Autodesk Inventor part; units mm, degrees
ref_plane "YZ Plane" through (0, 0, 0) normal (1, 0, 0) x (0, 1, 0)
ref_plane "XZ Plane" through (0, 0, 0) normal (0, 1, 0) x (-1, 0, 0)
ref_plane "XY Plane" through (0, 0, 0) normal (0, 0, 1) x (1, 0, 0)
sketch "スケッチ1" plane through (0, 0, 0) normal (0, 1, 0) x (-1, 0, 0)
  circle A0 centre (0, 0) radius 25
  circle A1 centre (0, 0) radius 30
  dimension "d0" = 50
  dimension "d1" = 60
extrude "押し出し1" add sketch "スケッチ1" along normal blind 60
sketch "スケッチ2" plane through (0, 0, 0) normal (0, 0, 1) x (1, 0, 0)
  line L0 (-5, 30.9364) -> (5, 30.9364)
  line L1 (5, 30.9364) -> (5, 22.9364)
  line L2 (5, 22.9364) -> (-5, 22.9364)
  line L3 (-5, 22.9364) -> (-5, 30.9364)
  line L4 (-5, 30.9364) -> (5, 22.9364) construction
  line L5 (5, 30.9364) -> (-5, 22.9364) construction
  point P0 (0, 0)
  point P1 (0, 26.9364)
  dimension "d4" = 10
  dimension "d5" = 8
extrude "押し出し2" cut sketch "スケッチ2" along normal mid plane 60
sketch "スケッチ3" plane through (0, 0, 0) normal (0, 0, 1) x (1, 0, 0)
  point P0 (0, 0)
sketch "スケッチ4" plane through (0, 0, 0) normal (0, 0, 1) x (1, 0, 0)
  line L0 (4, -5) -> (-4, -5)
  line L1 (-4, -5) -> (-4, 5)
  line L2 (-4, 5) -> (4, 5)
  line L3 (4, 5) -> (4, -5)
  line L4 (4, -5) -> (-4, 5) construction
  line L5 (-4, -5) -> (4, 5) construction
  point P0 (0, 0)
  dimension "d8" = 8
  dimension "d9" = 10
extrude "押し出し3" cut sketch "スケッチ4" along normal mid plane 60
properties part number "pipe"
Can you work these out from the model? Positions are in its coordinate system, mm. A direction names the side the tool comes from. Give positions to 0.01 mm unless a question says otherwise; leave off trailing zeros. Loops run counter-clockwise (first coordinate to the right, second up) from the corner with the lowest first, then second, coordinate; pieces in that order, holes last. Notation, with made-up numbers: (68.25, 73) -> (74.25, 73) arc R29 cw to (74.25, 97) -> close; hole circle Ø1 at (13.5, 53). An arc over 180 degrees is marked (long way). Use one line per item in the form item = value.
1) If we section it at C-C (x = -9): Please give me the cut outline in (y, z), plus the area to 3 significant figures.
Answers:
outline = (0, -28.62) -> (60, -28.62) -> (60, -23.32) -> (0, -23.32) -> close; (0, 23.32) -> (60, 23.32) -> (60, 28.62) -> (0, 28.62) -> close
area = 635 mm²
2) Will these pins go through, and if not, where does the flat tip stop? pin 1 (3 mm diameter, centred on x = -1, z = -27, fed in from -Y); pin 2 (12 mm diameter, centred on x = 22.5, y = 20, fed in from -Z); pin 3 (2 mm diameter, centred on y = 7.5, z = -4, fed in from +X); pin 4 (12 mm diameter, centred on y = 38.5, z = 4, fed in from -X).
Answers:
pin_1 = 5
pin_2 = -25.05
pin_3 = 29.85
pin_4 = -30
3) If we section it at D-D (y = 33): Please give me the cut outline in (x, z).
Answers:
outline = circle Ø60 at (0, 0); hole circle Ø50 at (0, 0)
4) If we section it at A-A (x = 0): Please give me the cut outline in (y, z), plus the area to 3 significant figures.
Answers:
outline = (5, -30) -> (22.94, -30) -> (22.94, -25) -> (5, -25) -> close; (5, 25) -> (22.94, 25) -> (22.94, 30) -> (5, 30) -> close; (30.94, -30) -> (60, -30) -> (60, -25) -> (30.94, -25) -> close; (30.94, 25) -> (60, 25) -> (60, 30) -> (30.94, 30) -> close
area = 470 mm²
5) I need wall thicknesses on line 1 along X through (y, z) = (41, 0); line 2 along Z through (x, y) = (-23, 7). Which ranges of each line are inside material? Lowest first, please.
Answers:
line_1 = -30 to -25, 25 to 30
line_2 = -19.26 to -9.8, 9.8 to 19.26
6) We'd pull the mould along Y, two halves only. Please class faces 1 (the face through (-25, 0, -4)), 2 (the face through (-4, 2, -27)), 3 (the face through (5, 27, -27)): released by +Y, released by -Y, zero draft, split by the parting line, or undercut.
Answers:
face_1 = released by -Y
face_2 = zero draft
face_3 = undercut
7) If we section it at B-B (z = 0): Please give me the cut outline in (x, y), plus the area to 3 significant figures.
Answers:
outline = (-30, 0) -> (-25, 0) -> (-25, 60) -> (-30, 60) -> close; (25, 0) -> (30, 0) -> (30, 60) -> (25, 60) -> close
area = 600 mm²
8) For faces 4 (the face through (7, 60, 25)), 5 (the face through (0, 22.936, 27)), 6 (the face through (4, 3, 27)), which set-ups out of +Z, -Z, +X, -X, +Y, -Y let a thin tool reach every point of the face, with its end or its side?
Answers:
face_4 = +Z, -Z, +X, -X, +Y
face_5 = +Z, -Z
face_6 = +Z, -Z, -Y
